Build history of the part. All positions in model axes, mm. Face numbers are marked on the shaded views. A direction names the side the tool comes from. Give positions to 0.01 mm unless a question says otherwise; leave off trailing zeros. Order: outer loops, then holes, each group sorted by start corner. A loop starts at its lowest first (then second) coordinate and runs counter-clockwise, first axis right, second up. Notation, with made-up numbers: (-39.75, 35) - (-22.75, 35) arc R7 ccw to (-22.75, 40) - close; hole circle Ø10 at (19, 25.5). An arc over 180 degrees is marked (long way). One line per item, written item: value.
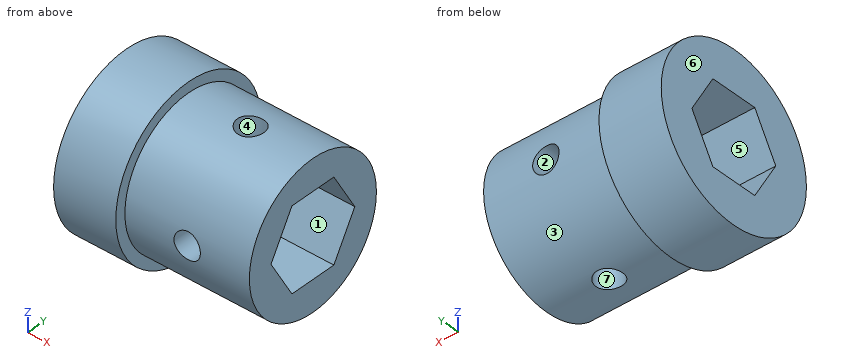
```python
from build123d import *

# Parameters (mm, degrees)
SKETCH1_R               = 11.1125
BOSS_EXTRUDE1_DEPTH     = 19.05
SKETCH2_R               = 12.7
BOSS_EXTRUDE2_DEPTH     = 9.525
CUT_EXTRUDE1_DEPTH      = 34.750712955
CUT_EXTRUDE2_DEPTH      = 27.181720723
CUT_EXTRUDE2_DEPTH_BACK = 27.181720723
SKETCH5_R               = 2.0193
CUT_EXTRUDE3_DEPTH      = 27.181720795
CUT_EXTRUDE3_DEPTH_BACK = 27.181720795
SKETCH6_R               = 2.0193


with BuildPart() as part:
    # Sketch1 → Boss-Extrude1 (new body)
    with BuildSketch(Plane(origin=(0, 0, 0), x_dir=(0, 0, -1), z_dir=(1, 0, 0))):
        with Locations(Location((0, 0, 0), (0, 0, 180))):
            Circle(SKETCH1_R)
    extrude(amount=BOSS_EXTRUDE1_DEPTH)

    # Sketch2 → Boss-Extrude2 (add)
    with BuildSketch(Plane.ZY):
        with Locations(Location((0, 0, 0), (0, 0, 180))):
            Circle(SKETCH2_R)
    extrude(amount=BOSS_EXTRUDE2_DEPTH)

    # Sketch4 → Cut-Extrude1 (cut, through all)
    with BuildSketch(Plane.ZY.offset(9.525)):
        Polygon((0, 7.332348419), (-6.35, 3.666174209), (-6.35, -3.666174209), (0, -7.332348419), (6.35, -3.666174209), (6.35, 3.666174209), align=None)
    extrude(amount=-CUT_EXTRUDE1_DEPTH, mode=Mode.SUBTRACT)

    # Sketch5 → Cut-Extrude2 (cut, two sides: drawn at the far end of the back side and taken through both)
    with BuildSketch(Plane.XY.offset(-CUT_EXTRUDE2_DEPTH_BACK)):
        with Locations((9.525, 0)):
            Circle(SKETCH5_R)
    extrude(amount=CUT_EXTRUDE2_DEPTH + CUT_EXTRUDE2_DEPTH_BACK, mode=Mode.SUBTRACT)

    # Sketch6 → Cut-Extrude3 (cut, two sides: drawn at the far end of the back side and taken through both)
    with BuildSketch(Plane(origin=(0, 0, 0), x_dir=(1, 0, 0), z_dir=(0, 1, 0)).offset(-CUT_EXTRUDE3_DEPTH_BACK)):
        with Locations(Location((9.525, 0, 0), (0, 0, 270))):
            Circle(SKETCH6_R)
    extrude(amount=CUT_EXTRUDE3_DEPTH + CUT_EXTRUDE3_DEPTH_BACK, mode=Mode.SUBTRACT)


solid = part.part
```
(1) Slice it at D-D, the plane z = 1. Give the cut face in (x, y) (3 decimals), and give its area (3 significant figures).
Completed:
outline: (-9.525, -12.661) - (0, -12.661) - (0, -11.067) - (7.771, -11.067) - (7.771, -6.755) - (-9.525, -6.755) - close; (-9.525, 6.755) - (7.771, 6.755) - (7.771, 11.067) - (0, 11.067) - (0, 12.661) - (-9.525, 12.661) - close; (11.279, -11.067) - (19.05, -11.067) - (19.05, -6.755) - (11.279, -6.755) - close; (11.279, 6.755) - (19.05, 6.755) - (19.05, 11.067) - (11.279, 11.067) - close
area: 247 mm²
(2) 3-axis set-ups, long thin cutter, end or side, ignore diameter. For the marked faces 1, 2 and 3: which of +Z, -Z, +X, -X, +Y, -Y reach the whole face in a straight line?
Completed:
face 1: +X, -X
face 2: +Y, -Y
face 3: +X
(3) Pull direction X, two halves, no side cores. Call the marked faces 4, 5, 6 and 7: +X half, -X half, draft (parallel to the pull), parting line (faces both ways), or undercut.
Completed:
face 4: undercut
face 5: draft
face 6: -X half
face 7: undercut
(4) Pin check, flat tips, straight feed: P1, Ø5.5, axis at x = 9.525, y = 0, coming from the -Z side; P2, Ø4, axis at x = -6.5, z = -7.5, coming from the -Y side; P3, Ø2, axis at x = 5, y = 9, coming from the +Z side. Stop position of each tip, or through.
Completed:
P1: z = -11.11
P2: y = -11.45
P3: z = 7.71
(5) Slice it at C-C, the plane z = -4. Give the cut face in (x, y) (3 decimals).
Completed:
outline: (-9.525, -12.054) - (0, -12.054) - (0, -10.368) - (19.05, -10.368) - (19.05, -5.023) - (-9.525, -5.023) - close; (-9.525, 5.023) - (19.05, 5.023) - (19.05, 10.368) - (0, 10.368) - (0, 12.054) - (-9.525, 12.054) - close
(6) Drill centre lines: line 1 (X direction, y = 0, z = 9.25) (3 decimals); line 2 (Y direction, x = -5.25, z = -2.75); line 3 (Y direction, x = 14, z = 3.75). Where is each one in solid material? Low to high.
Completed:
line 1: -9.525 to 7.506, 11.544 to 19.05
line 2: -12.4 to -5.74, 5.74 to 12.4
line 3: -10.46 to -5.17, 5.17 to 10.46
(7) Slice it at B-B, the plane y = 0. Count the separate pieces of the cut face and the enclosed holes in it, and give its area (3 significant figures).
Completed:
separate pieces: 4
enclosed holes: 0
area: 264 mm²
